Here's how the part is built. I have some questions about the finished solid (model axes, mm). A direction names the side the tool comes from. Coordinates: 2 decimals unless noted, no trailing zeros. Write each loop counter-clockwise with the first axis right and the second up, starting at its lowest first coordinate (ties: lowest second). Pieces come first, ordered by that corner, then holes.
(1) For pin 1 Ø2.5 at (y, z) = (10, 14.2) entering from +X; pin 2 Ø4 at (x, y) = (14.5, 8.5) entering from +Z, each with a flat end and sliding along its axis, tell me the tip position at first contact or that it passes through.
(2) Imagine slicing it at B-B, the plane y = 4. List the corners of the cut face in (x, z) for me.
(3) Imagine slicing it at A-A, the plane z = 14.2. List the corners of the cut face in (x, y) for me, plus the area to 3 significant figures.
(4) Which directions (+Z, -Z, +X, -X, +Y, -Y) give clear straight access to the entire face, cutting with the end or side of a thin tool? Please do faces 1 (the cylindrical face through (1.12, 10.09, 22.35)), 2 (the flat face through (17, 10, 2.2)).
(5) Thinking about a two-plate mould opening in Y: for faces 3 (the cylindrical face through (33.32, 10.09, 22.35)), 4 (the cylindrical face through (29.794, 9.86, 4.481)), 5 (the cylindrical face through (33.285, 17.594, 26.919)), which applies, released by +Y, released by -Y, zero draft, split by the parting line, or undercut?
(6) Please list where these lines run through material, in increasing order: probe 1 along X at (y, z) = (9.5, 10); probe 2 along Y at (x, z) = (32.7, 14.2); probe 3 along X at (y, z) = (1.75, 4).
(7) Imagine slicing it at C-C, the plane y = 10. State how many separate pieces and enclosed holes the cut face has, plus the area to 3 significant figures.
(8) Imagine slicing it at D-D, the plane x = 23.5. List the corners of the cut face in (y, z) for me, plus the area to 3 significant figures.
Autodesk Inventor part; units mm, degrees
ref_plane "YZ Plane" through (0, 0, 0) normal (1, 0, 0) x (0, 1, 0)
ref_plane "XZ Plane" through (0, 0, 0) normal (0, 1, 0) x (-1, 0, 0)
ref_plane "XY Plane" through (0, 0, 0) normal (0, 0, 1) x (1, 0, 0)
sketch "Esquisse1" plane through (0, 0, 0) normal (0, 0, 1) x (1, 0, 0)
  line L0 (0, 0) -> (34.4, 0)
  line L1 (34.4, 0) -> (34.4, 20)
  line L2 (34.4, 20) -> (0, 20)
  line L3 (0, 20) -> (0, 0)
  dimension "d0" = 34.4
  dimension "d1" = 20
extrude "Extrusion1" add sketch "Esquisse1" along normal blind 2.2
sketch "Esquisse2" plane through (0, 0, 2.2) normal (0, 0, 1) x (1, 0, 0)
  line L0 (0, 0) -> (34.4, 0)
  line L1 (34.4, 20) -> (0, 20)
  line L2 (0, 20) -> (0, 0)
  line L3 (0, 20) -> (2.2, 20)
  line L4 (2.2, 20) -> (2.2, 0)
  line L5 (2.2, 0) -> (0, 0)
  line L6 (0, 0) -> (0, 20)
  line L7 (17.2, 20) -> (17.2, 0) construction
  line L8 (34.4, 20) -> (32.2, 20)
  line L9 (32.2, 20) -> (32.2, 0)
  line L10 (32.2, 0) -> (34.4, 0)
  line L11 (34.4, 0) -> (34.4, 20)
  dimension "d4" = 2.2
extrude "Extrusion2" add sketch "Esquisse2" along normal blind 27 contours L2 L1 L4 L0 | L9 L1 L11 L0
sketch "Esquisse3" plane through (34.4, 0, 0) normal (1, 0, 0) x (0, 0, -1)
  line L0 (0, 0) -> (0, 20) construction
  line L1 (-29.2, 0) -> (-29.2, 20) construction
  line L2 (-29.2, 10) -> (0, 10) construction
  circle A0 centre (-20.2, 10) radius 2.15
  line L3 (-20.2, 10) -> (-20.2, 15.2246) construction
  circle A1 centre (-14.2, 10) radius 2.15
  circle A2 centre (-26.2, 10) radius 2.15
  circle A3 centre (-20.2, 10) radius 2.15
  circle A4 centre (-20.2, 16) radius 2.15
  circle A5 centre (-20.2, 4) radius 2.15
  circle A6 centre (-20.2, 10) radius 2.15
  dimension "d7" = 9
  dimension "d8" = 4.3
  dimension "d11" = 6
  dimension "d14" = 6
  dimension "d19" = 6
  dimension "d22" = 6
extrude "Extrusion3" cut sketch "Esquisse3" against normal through all
fillet "Congé1" radius 8 4 edges at (33.3, 20, 29.2) (1.1, 20, 29.2) (1.1, 0, 29.2) (33.3, 0, 29.2)
fillet "Congé2" radius 8 4 edges at (2.2, 10, 2.2) (0, 10, 0) (34.4, 10, 0) (32.2, 10, 2.2)
equation "\"d2\" = UDepth"
equation "\"d4\" = Depth"
equation "\"d8\" = Holes"
equation "\"d28\" = URound"
equation "\"Depth\" = 2.2"
equation "\"Holes\" = 4.3"
equation "\"UDepth\" = Depth"
equation "\"USize\" = 5"
equation "\"URound\" = 8"
properties part number "U"
Recorded:
1. pin 1: passes through
1. pin 2: stops at z = 2.2
2. outline: (0, 8) arc R8 ccw to (8, 0) - (26.4, 0) arc R8 ccw to (34.4, 8) - (34.4, 18.05) - (32.2, 18.05) - (32.2, 10.2) arc R8 cw to (24.2, 2.2) - (10.2, 2.2) arc R8 cw to (2.2, 10.2) - (2.2, 18.05) - (0, 18.05) - close; (0, 22.35) - (2.2, 22.35) - (2.2, 28.13) - (0, 28.13) - close; (32.2, 22.35) - (34.4, 22.35) - (34.4, 28.13) - (32.2, 28.13) - close
3. outline: (0, 0) - (2.2, 0) - (2.2, 7.85) - (0, 7.85) - close; (0, 12.15) - (2.2, 12.15) - (2.2, 20) - (0, 20) - close; (32.2, 0) - (34.4, 0) - (34.4, 7.85) - (32.2, 7.85) - close; (32.2, 12.15) - (34.4, 12.15) - (34.4, 20) - (32.2, 20) - close
3. area: 69.1 mm2
4. face 1: +X, -X
4. face 2: +Z, +Y, -Y
5. face 3: undercut
5. face 4: zero draft
5. face 5: released by +Y
6. probe 1: x = 0 to 2.2, 32.2 to 34.4
6. probe 2: y = 0 to 7.85, 12.15 to 20
6. probe 3: x = 1.07 to 5.14, 29.26 to 33.33
7. separate pieces: 7
7. enclosed holes: 0
7. area: 138 mm2
8. outline: (0, 0) - (20, 0) - (20, 2.2) - (0, 2.2) - close
8. area: 44.0 mm2
